```python
from build123d import *
from build123d.topology import SkipClean

# Parameters (mm, degrees)
SKETCH_1_W               = 16
SKETCH_1_H               = 10.345
SKETCH_4_W               = 2
SKETCH_4_H               = 1.101020514
CUT_EXTRUDE_1_DEPTH      = 27.961788702
CUT_EXTRUDE_2_REACH      = 28.962
PATTERN_CIRCULAR_3_COUNT = 20
EXTRUDE_START            = 2
SKETCH_7_R               = 17
EXTRUDE_1_DEPTH          = 2
SKETCH_8_R               = 17
EXTRUDE_2_DEPTH          = 2
EXTRUDE_START_2          = -20
EXTRUDE_3_DEPTH          = 20


with BuildPart() as part:
    # 草图1 → 旋转1 (revolve)
    with BuildSketch(Plane.XY, mode=Mode.PRIVATE) as revolve_1_sk:
        with Locations((8, 10.1725)):
            Rectangle(SKETCH_1_W, SKETCH_1_H)
    revolve(revolve_1_sk.sketch.rotate(Axis((0, 0, 0), (1, 0, 0)), 90), axis=Axis((0, 0, 0), (1, 0, 0)))

    # 草图4 → 切除-拉伸1 (cut, through all)
    with BuildSketch(Plane.ZY):
        with Locations((0, 5.449489743)):
            Rectangle(SKETCH_4_W, SKETCH_4_H)
    extrude(amount=-CUT_EXTRUDE_1_DEPTH, mode=Mode.SUBTRACT)

    # 草图6 → 切除-拉伸2 (cut, up to next)
    with BuildSketch(Plane(origin=(0, 0, 0), x_dir=(0, 0, -1), z_dir=(1, 0, 0)), mode=Mode.PRIVATE) as cut_extrude_2_sk1:
        with BuildLine():
            Line((1.29350436, 14.889411229), (1.049088646, 14.114223621))
            ThreePointArc((1.049088646, 14.114223621), (0, 13.345), (-1.049088646, 14.114223621))
            Line((-1.049088646, 14.114223621), (-1.29350436, 14.889411229))
            ThreePointArc((-1.29350436, 14.889411229), (-1.499322423, 15.159221505), (-1.829991088, 15.235490068))
            ThreePointArc((-1.829991088, 15.235490068), (-2.077964077, 15.203653847), (-2.325385479, 15.167781887))
            Line((-2.325385479, 15.167781887), (-2.810603409, 16.706696553))
            ThreePointArc((-2.810603409, 16.706696553), (0, 16.941463964), (2.810603409, 16.706696553))
            Line((2.810603409, 16.706696553), (2.325385479, 15.167781887))
            ThreePointArc((2.325385479, 15.167781887), (2.077964077, 15.203653847), (1.829991088, 15.235490068))
            ThreePointArc((1.829991088, 15.235490068), (1.499322423, 15.159221505), (1.29350436, 14.889411229))
        make_face()
    cut_extrude_2_tool1 = extrude(cut_extrude_2_sk1.sketch, amount=CUT_EXTRUDE_2_REACH, mode=Mode.PRIVATE) & part.part
    cut_extrude_2 = cut_extrude_2_tool1.solids().sort_by_distance((0, 15.551967, 0))[0]
    add(cut_extrude_2, mode=Mode.SUBTRACT)

    # 阵列(圆周)3: 切除-拉伸2 ×20 about axis
    pattern_circular_3_axis = Axis((0, 0, 0), (1, 0, 0))
    for i in range(1, PATTERN_CIRCULAR_3_COUNT):
        add(cut_extrude_2.rotate(pattern_circular_3_axis, i * 360 / PATTERN_CIRCULAR_3_COUNT), mode=Mode.SUBTRACT)

    # 草图7 → 凸台-拉伸1 (add)
    with BuildSketch(Plane.ZY.offset(EXTRUDE_START)):
        Circle(SKETCH_7_R)
        with BuildLine():
            Line((-1, 6), (-1, 4.898979486))
            ThreePointArc((-1, 4.898979486), (0, -5), (1, 4.898979486))
            Line((1, 4.898979486), (1, 6))
            Line((1, 6), (-1, 6))
        make_face(mode=Mode.SUBTRACT)
    extrude(amount=-EXTRUDE_1_DEPTH)

    # 草图8 → 凸台-拉伸2 (add)
    with BuildSketch(Plane(origin=(16, 0, 0), x_dir=(0, 0, -1), z_dir=(1, 0, 0))):
        with Locations(Location((0, 0, 0), (0, 0, 180))):
            Circle(SKETCH_8_R)
        with BuildLine():
            Line((1, 6), (1, 4.898979486))
            ThreePointArc((1, 4.898979486), (0, -5), (-1, 4.898979486))
            Line((-1, 4.898979486), (-1, 6))
            Line((-1, 6), (1, 6))
        make_face(mode=Mode.SUBTRACT)
    extrude(amount=EXTRUDE_2_DEPTH)

    # 草图9 → 凸台-拉伸3 (add)
    with SkipClean():  # the faces are left unmerged after this step: merging them gives an invalid solid
        with BuildSketch(Plane(origin=(18, 0, 0), x_dir=(0, 0, -1), z_dir=(1, 0, 0)).offset(EXTRUDE_START_2)):
            with BuildLine():
                Line((-1, 4.898979486), (-1, 6))
                Line((-1, 6), (1, 6))
                Line((1, 6), (1, 4.898979486))
                ThreePointArc((1, 4.898979486), (0, 5), (-1, 4.898979486))
            make_face()
        extrude(amount=EXTRUDE_3_DEPTH)


solid = part.part
```
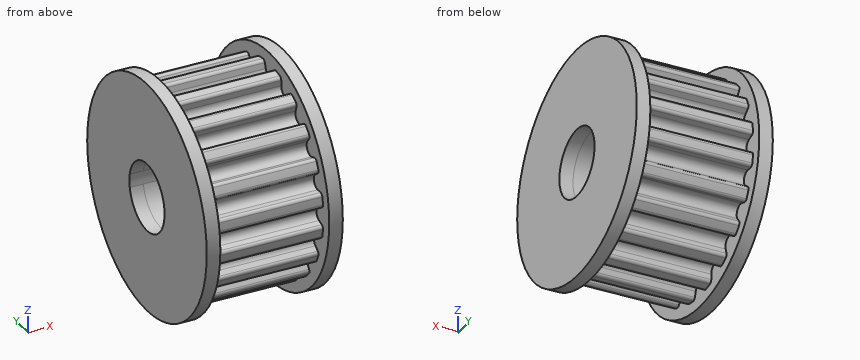
Build history of the part. All positions in model axes, mm. Give positions to 0.01 mm unless a question says otherwise; leave off trailing zeros. Order: outer loops, then holes, each group sorted by start corner. A loop starts at its lowest first (then second) coordinate and runs counter-clockwise, first axis right, second up. Notation, with made-up numbers: M -19.5,16 L 7.5,16 A20 ccw 7.5,26 Z; hole C 43,41.5 d2. An arc over 180 degrees is marked long. Return JSON: item names as keys, results as strings.
Q1. Wall check: probe 1 along Z at (x, y) = (3.75, 0) (3 decimals); probe 2 along X at (y, z) = (13.5, 10); probe 3 along Y at (x, z) = (7.75, 10). Give the ranges that are in metal, low to high. Write a range as from..to.
Answer list:
{"probe 1": "z = -13.345..-5, 5..13.345", "probe 2": "x = -2..0, 16..18", "probe 3": "y = -11.37..11.37"}
Q2. Flat gauge pins, fed straight in: pin 1 (8 mm diameter, centred on x = 10.5, z = 8, fed in from +Y); pin 2 (3 mm diameter, centred on x = 0.5, z = -2.5, fed in from -Y); pin 3 (3 mm diameter, centred on x = 10, y = -9, fed in from -Z). Where does each tip first touch, or does it go through?
Answer list:
{"pin 1": "stops at y = 13.97", "pin 2": "stops at y = -16.97", "pin 3": "stops at z = -13.39"}
Q3. Band-saw the part on D-D (y = 8.5). Give the cut face in (x, z), then the cut area to 3 significant figures.
Answer list:
{"outline": "M -2,-14.72 L 0,-14.72 L 0,-10.59 L 16,-10.59 L 16,-14.72 L 18,-14.72 L 18,14.72 L 16,14.72 L 16,10.59 L 0,10.59 L 0,14.72 L -2,14.72 Z", "area": "457 mm^2"}
Q4. Band-saw the part on A-A (y = 0). Give the cut face in (x, z) (3 decimals), then the cut area to 3 significant figures.
Answer list:
{"outline": "M -2,-17 L 0,-17 L 0,-13.345 L 16,-13.345 L 16,-17 L 18,-17 L 18,-5 L -2,-5 Z; M -2,5 L 18,5 L 18,17 L 16,17 L 16,13.345 L 0,13.345 L 0,17 L -2,17 Z", "area": "363 mm^2"}
Q5. Band-saw the part on C-C (x = 16.75). Give the cut face in (y, z).
Answer list:
{"outline": "C 0,0 d34; hole C 0,0 d10"}
